Check sheet for the modelled part. Datum: model origin and axes. Units: mm. A direction names the side the tool comes from. Give positions to 0.01 mm unless a question says otherwise; leave off trailing zeros. Write each loop counter-clockwise with the first axis right and the second up, starting at its lowest first coordinate (ties: lowest second). Pieces come first, ordered by that corner, then holes. Notation, with made-up numbers: (86.5, -6) -> (125.5, -6) arc R33 ccw to (125.5, 25) -> close; hole circle Ø4 at (86, 33). An arc over 180 degrees is marked (long way). Use a Markdown table: item, result. Add a question column.
1. Cross-section at B-B (x = 3.5). Enter the section's corners in (y, z).
2. Release check for a two-part mould opening along Z. For faces 1 (the flat face through (-30, 3, 20)), 2 (the flat face through (0, 3, 3)), 3 (the flat face through (-1, 5, 0)), 4 (the flat face through (30, 2, -20)) record: released by +Z, released by -Z, zero draft, split by the parting line, or undercut.
3. Cross-section at D-D (z = 21). Enter the section's corners in (x, y).
4. Gauge pin test, flat ends, axial feed: P1, Ø2, axis at x = 13.5, z = -15, coming from the +Y side; P2, Ø1.5, axis at y = 2.5, z = -11.5, coming from the +X side; P3, Ø1.5, axis at y = 2.5, z = 7, coming from the -X side. Record the tip position at first contact, or that the pin passes through.
5. Cross-section at C-C (x = 31). Enter the section's corners in (y, z).
6. Scan lines: probe 1 along Z at (x, y) = (0, 3); probe 2 along Z at (x, y) = (-15, 0.7); probe 3 along Z at (x, y) = (-10, 3.65). Record each from-to range of solid material in increasing order. Write a range as [from, to].
7. Cross-section at A-A (y = 0.9). Enter the section's corners in (x, z), then the cut area to 3 significant figures.
8. Set-up check for faces 5 (the flat face through (-8.78, 2.54, 14.93)), 6 (the flat face through (-15, 2, -17)), 7 (the flat face through (-42.5, 2, -16)): record each of +Z, -Z, +X, -X, +Y, -Y from which the full face is reachable in a straight line by a thin tool's end or side.
from build123d import *

# Parameters (mm, degrees)
SKETCH1_W           = 85
SKETCH1_H           = 65
BOSS_EXTRUDE1_DEPTH = 5
CUT_EXTRUDE1_DEPTH  = 46
CUT_EXTRUDE2_DEPTH  = 46
SKETCH5_W           = 45.682853102
SKETCH5_H           = 6
BOSS_EXTRUDE3_DEPTH = 5
SKETCH6_R           = 3.6
CUT_EXTRUDE3_DEPTH  = 3
CUT_EXTRUDE4_DEPTH  = 5
FILLET1_R           = 20


with BuildPart() as part:
    # Sketch1 → Boss-Extrude1 (new body)
    with BuildSketch(Plane(origin=(0, 0, 0), x_dir=(1, 0, 0), z_dir=(0, 1, 0))):
        Rectangle(SKETCH1_W, SKETCH1_H)
    extrude(amount=BOSS_EXTRUDE1_DEPTH)

    # Sketch3 → Cut-Extrude1 (cut)
    with BuildSketch(Plane(origin=(0, 5, 0), x_dir=(1, 0, 0), z_dir=(0, 1, 0))):
        with BuildLine():
            ThreePointArc((-13.4, 15), (-16.13137085, 16.13137085), (-15, 13.4))
            Line((-15, 13.4), (-15, 15))
            Line((-15, 15), (-13.4, 15))
        make_face()
        with BuildLine():
            Line((-15, 15), (-15, 13.4))
            ThreePointArc((-15, 13.4), (-13.86862915, 13.86862915), (-13.4, 15))
            Line((-13.4, 15), (-15, 15))
        make_face()
        with BuildLine():
            ThreePointArc((-13.4, 15), (-16.13137085, 16.13137085), (-15, 13.4))
            Line((-15, 13.4), (-15, 15))
            Line((-15, 15), (-13.4, 15))
        make_face()
        with BuildLine():
            Line((-15, 15), (-15, 13.4))
            ThreePointArc((-15, 13.4), (-13.86862915, 13.86862915), (-13.4, 15))
            Line((-13.4, 15), (-15, 15))
        make_face()
        with BuildLine():
            ThreePointArc((13.4, 15), (13.86862915, 13.86862915), (15, 13.4))
            Line((15, 13.4), (15, 15))
            Line((15, 15), (13.4, 15))
        make_face()
        with BuildLine():
            Line((15, 15), (15, 13.4))
            ThreePointArc((15, 13.4), (16.13137085, 13.86862915), (16.6, 15))
            ThreePointArc((16.6, 15), (15, 16.6), (13.4, 15))
            Line((13.4, 15), (15, 15))
        make_face()
        with BuildLine():
            ThreePointArc((13.4, 15), (13.86862915, 13.86862915), (15, 13.4))
            Line((15, 13.4), (15, 15))
            Line((15, 15), (13.4, 15))
        make_face()
        with BuildLine():
            Line((15, 15), (15, 13.4))
            ThreePointArc((15, 13.4), (16.13137085, 13.86862915), (16.6, 15))
            ThreePointArc((16.6, 15), (15, 16.6), (13.4, 15))
            Line((13.4, 15), (15, 15))
        make_face()
        with BuildLine():
            Line((-15, -13.4), (-15, -15))
            Line((-15, -15), (-13.4, -15))
            ThreePointArc((-13.4, -15), (-13.86862915, -13.86862915), (-15, -13.4))
        make_face()
        with BuildLine():
            Line((-13.4, -15), (-15, -15))
            Line((-15, -15), (-15, -13.4))
            ThreePointArc((-15, -13.4), (-16.13137085, -16.13137085), (-13.4, -15))
        make_face()
        with BuildLine():
            Line((-15, -13.4), (-15, -15))
            Line((-15, -15), (-13.4, -15))
            ThreePointArc((-13.4, -15), (-13.86862915, -13.86862915), (-15, -13.4))
        make_face()
        with BuildLine():
            Line((-13.4, -15), (-15, -15))
            Line((-15, -15), (-15, -13.4))
            ThreePointArc((-15, -13.4), (-16.13137085, -16.13137085), (-13.4, -15))
        make_face()
        with BuildLine():
            ThreePointArc((15, -13.4), (13.86862915, -13.86862915), (13.4, -15))
            Line((13.4, -15), (15, -15))
            Line((15, -15), (15, -13.4))
        make_face()
        with BuildLine():
            Line((15, -15), (13.4, -15))
            ThreePointArc((13.4, -15), (15, -16.6), (16.6, -15))
            ThreePointArc((16.6, -15), (16.13137085, -13.86862915), (15, -13.4))
            Line((15, -13.4), (15, -15))
        make_face()
        with BuildLine():
            ThreePointArc((15, -13.4), (13.86862915, -13.86862915), (13.4, -15))
            Line((13.4, -15), (15, -15))
            Line((15, -15), (15, -13.4))
        make_face()
        with BuildLine():
            Line((15, -15), (13.4, -15))
            ThreePointArc((13.4, -15), (15, -16.6), (16.6, -15))
            ThreePointArc((16.6, -15), (16.13137085, -13.86862915), (15, -13.4))
            Line((15, -13.4), (15, -15))
        make_face()
    extrude(amount=-CUT_EXTRUDE1_DEPTH, mode=Mode.SUBTRACT)

    # Sketch4 → Cut-Extrude2 (cut)
    with BuildSketch(Plane(origin=(0, 5, 0), x_dir=(1, 0, 0), z_dir=(0, 1, 0))):
        Polygon((0, -20), (17.320508076, -10), (17.320508076, 10), (0, 20), (-17.320508076, 10), (-17.320508076, -10), align=None)
    extrude(amount=-CUT_EXTRUDE2_DEPTH, mode=Mode.SUBTRACT)

    # Sketch5 → Boss-Extrude3 (add)
    with BuildSketch(Plane(origin=(0, 5, 0), x_dir=(1, 0, 0), z_dir=(0, 1, 0))):
        Rectangle(SKETCH5_W, SKETCH5_H)
    extrude(amount=-BOSS_EXTRUDE3_DEPTH)

    # Sketch6 → Cut-Extrude3 (cut)
    with BuildSketch(Plane(origin=(0, 5, 0), x_dir=(1, 0, 0), z_dir=(0, 1, 0))):
        with Locations((-15, 15)):
            Circle(SKETCH6_R)
        with Locations((15, 15)):
            Circle(SKETCH6_R)
        with Locations((-15, -15)):
            Circle(SKETCH6_R)
        with Locations((15, -15)):
            Circle(SKETCH6_R)
    extrude(amount=-CUT_EXTRUDE3_DEPTH, mode=Mode.SUBTRACT)

    # Sketch7 → Cut-Extrude4 (cut, symmetric)
    with BuildSketch(Plane(origin=(0, 5, 0), x_dir=(1, 0, 0), z_dir=(0, 1, 0))):
        Polygon((17.5, 32.5), (42.5, 7.5), (42.5, 32.5), align=None)
        Polygon((-42.5, -32.5), (-17.5, -32.5), (-42.5, -7.5), align=None)
    extrude(amount=CUT_EXTRUDE4_DEPTH, both=True, mode=Mode.SUBTRACT)

    # Fillet1
    fillet1_edges = [part.edges().sort_by_distance(p)[0] for p in [
        (42.5, 2.5, -7.5),
        (17.5, 2.5, -32.5),
        (-17.5, 2.5, 32.5),
        (-42.5, 2.5, 7.5),
    ]]
    fillet(fillet1_edges, radius=FILLET1_R)


solid = part.part
Worked answers:
| question | item | result |
|---|---|---|
| 1 | outline | (0, -32.5) -> (5, -32.5) -> (5, -17.98) -> (0, -17.98) -> close; (0, -3) -> (5, -3) -> (5, 3) -> (0, 3) -> close; (0, 17.98) -> (5, 17.98) -> (5, 32.5) -> (0, 32.5) -> close |
| 2 | face 1 | released by +Z |
| 2 | face 2 | undercut |
| 2 | face 3 | zero draft |
| 2 | face 4 | released by -Z |
| 3 | outline | (-29, 0) -> (42.5, 0) -> (42.5, 5) -> (-29, 5) -> close |
| 4 | P1 | stops at y = 2 |
| 4 | P2 | stops at x = 38.84 |
| 4 | P3 | stops at x = -41.22 |
| 5 | outline | (0, -19) -> (5, -19) -> (5, 32.5) -> (0, 32.5) -> close |
| 6 | probe 1 | z = [-32.5, -20], [-3, 3], [20, 32.5] |
| 6 | probe 2 | z = [-32.5, -16.6], [-13.4, -11.34], [-3, 3], [11.34, 13.4], [16.6, 31.65] |
| 6 | probe 3 | z = [-32.5, -14.23], [-3, 3], [14.23, 32.48] |
| 7 | outline | (-42.5, -32.5) -> (9.22, -32.5) arc R20 ccw to (23.36, -26.64) -> (36.64, -13.36) arc R20 ccw to (42.5, 0.78) -> (42.5, 32.5) -> (-9.22, 32.5) arc R20 ccw to (-23.36, 26.64) -> (-36.64, 13.36) arc R20 ccw to (-42.5, -0.78) -> close; hole (-17.32, -10) -> (0, -20) -> (17.32, -10) -> (17.32, -3) -> (-17.32, -3) -> close; hole (-17.32, 3) -> (17.32, 3) -> (17.32, 10) -> (0, 20) -> (-17.32, 10) -> close; hole circle Ø3.2 at (-15, -15); hole circle Ø3.2 at (-15, 15); hole circle Ø3.2 at (15, -15); hole circle Ø3.2 at (15, 15) |
| 7 | area | 4,000 mm² |
| 8 | face 5 | +Y, -Y |
| 8 | face 6 | +Y |
| 8 | face 7 | +Z, -Z, -X, +Y, -Y |
